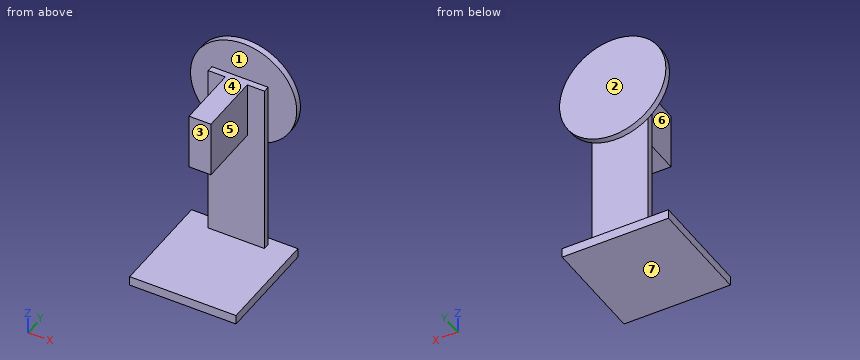
from build123d import *

# Parameters (mm, degrees)
F0_W      = 215.9
F0_H      = 215.9
F1_DEPTH  = 19.05
F3_W      = 114.3
F3_H      = 12.7
F4_DEPTH  = 355.6
F5_W      = 44.45
F5_H      = 127
F6_DEPTH  = 114.3
F9_R      = 6.35
F10_DEPTH = 12.7
F11_R     = 107.95
F12_DEPTH = 12.7


# Not quite as in the source:
# - a feature of the source that left no trace in its solid (it failed there, or was rolled back) is left out


with BuildPart() as f1:
    # F0 (on Top) → F1 (new body)
    with BuildSketch(Plane.XY):
        Rectangle(F0_W, F0_H)
    extrude(amount=F1_DEPTH)

    # F3 (on face) → F4 (join)
    with BuildSketch(Plane.XY.offset(19.05)):
        with Locations((0, 85.1799877524)):
            Rectangle(F3_W, F3_H)
    extrude(amount=F4_DEPTH)

    # F5 (on face) → F6 (join)
    with BuildSketch(Plane.XY.offset(374.65)):
        with Locations((0, 15.3299877524)):
            Rectangle(F5_W, F5_H)
    extrude(amount=-F6_DEPTH)

    # F9 (on face) → F10 (join)
    with BuildSketch(Plane(origin=(0, 91.5299877524, 0), x_dir=(-1, 0, 0), z_dir=(0, 1, 0))):
        with Locations((0, 332.823485136)):
            Circle(F9_R)
    extrude(amount=F10_DEPTH)

    # F11 (on face) → F12 (join)
    with BuildSketch(Plane(origin=(0, 104.2299877524, 0), x_dir=(-1, 0, 0), z_dir=(0, 1, 0))):
        with Locations((0, 332.823485136)):
            Circle(F11_R)
    extrude(amount=F12_DEPTH)


solid = f1.part
Part model, mm, in its own coordinate system. Face numbers are marked on the shaded views. A direction names the side the tool comes from. Coordinates: 2 decimals unless noted, no trailing zeros. Order: outer loops, then holes, each group sorted by start corner. A loop starts at its lowest first (then second) coordinate and runs counter-clockwise, first axis right, second up.
(1) Pull direction Y, two halves, no side cores. Call the marked faces 1, 2, 3 and 4: pulls with the +Y half, pulls with the -Y half, needs draft (parallel to the pull), parting line crosses it, or undercut.
Check sheet entries:
face 1: undercut
face 2: pulls with the +Y half
face 3: pulls with the -Y half
face 4: needs draft
(2) Slice it at D-D, the plane z = 387. Write the cut outline in (x, y), and give its area (3 significant figures).
Check sheet entries:
outline: (-93.37, 104.23) - (93.37, 104.23) - (93.37, 116.93) - (-93.37, 116.93) - close
area: 2,370 mm2
(3) Probe L1, parallel to Y at x = -14, z = 274.5; L2, parallel to Y at x = 36, z = 133.5; L3, parallel to Z at x = 30, y = -63.5. List the from-to ranges inside material, lowest first.
Check sheet entries:
L1: y = -48.17 to 91.53, 104.23 to 116.93
L2: y = 78.83 to 91.53
L3: z = 0 to 19.05
(4) Slice it at C-C, the plane z = 92. Write the cut outline in (x, y).
Check sheet entries:
outline: (-57.15, 78.83) - (57.15, 78.83) - (57.15, 91.53) - (-57.15, 91.53) - close
(5) Pin check, flat tips, straight feed: pin 1 Ø6 at (x, y) = (-58.5, 5.5) entering from -Z; pin 2 Ø4 at (y, z) = (-28, 265) entering from +X (3 decimals); pin 3 Ø4 at (y, z) = (83, 217) entering from -X; pin 4 Ø5 at (x, y) = (77.5, 13) entering from +Z. Stop position of each tip, or through.
Check sheet entries:
pin 1: stops at z = 0
pin 2: stops at x = 22.225
pin 3: stops at x = -57.15
pin 4: stops at z = 19.05
(6) Tool access for the marked faces 5, 6 and 7: list every direction of +Z, -Z, +X, -X, +Y, -Y with a clear straight run to the whole face (end or side of a thin tool).
Check sheet entries:
face 5: +Z, +X, -Y
face 6: +Z, -X, -Y
face 7: -Z, +X, -X, +Y, -Y
(7) Slice it at A-A, the plane y = -22.5. Write the cut outline in (x, z) (3 decimals).
Check sheet entries:
outline: (-107.95, 0) - (107.95, 0) - (107.95, 19.05) - (-107.95, 19.05) - close; (-22.225, 260.35) - (22.225, 260.35) - (22.225, 374.65) - (-22.225, 374.65) - close
(8) Slice it at B-B, the plane x = 14.5. Write the cut outline in (y, z), and give its area (3 significant figures).
Check sheet entries:
outline: (-107.95, 0) - (107.95, 0) - (107.95, 19.05) - (91.53, 19.05) - (91.53, 374.65) - (-48.17, 374.65) - (-48.17, 260.35) - (78.83, 260.35) - (78.83, 19.05) - (-107.95, 19.05) - close; (104.23, 225.85) - (116.93, 225.85) - (116.93, 439.8) - (104.23, 439.8) - close
area: 25,900 mm2
